For this review, take the finished solid that the model builds, in its own axes (mm). Coordinates: 2 decimals unless noted, no trailing zeros. Write each loop counter-clockwise with the first axis right and the second up, starting at its lowest first coordinate (ties: lowest second). Pieces come first, ordered by that corner, then holes. Notation, with made-up numbers: M -23.5,88 L 8.5,88 A15 cw 8.5,111 Z; hole C 4,-30.5 d2. An arc over 180 degrees is marked long. One line per question, with ' | ' between items.
from build123d import *

# Parameters (mm, degrees)
SKETCH1_R                                      = 1.7
BOSS_EXTRUDE1_DEPTH                            = 1.5875
SKETCH2_R                                      = 9
CUT_EXTRUDE1_DEPTH                             = 2.5875
CSK_FOR_M3_FLAT_HEAD_MACHINE_SCREW1_AT_2_COUNT = 2
CSK_FOR_M3_FLAT_HEAD_MACHINE_SCREW1_AT_2_PITCH = 11.799694945
CSK_FOR_M3_FLAT_HEAD_MACHINE_SCREW1_AT_3_COUNT = 2
CSK_FOR_M3_FLAT_HEAD_MACHINE_SCREW1_AT_3_PITCH = 38.059706694
CSK_FOR_M3_FLAT_HEAD_MACHINE_SCREW1_AT_4_COUNT = 2
CSK_FOR_M3_FLAT_HEAD_MACHINE_SCREW1_AT_4_PITCH = 65.441137915
CSK_FOR_M3_FLAT_HEAD_MACHINE_SCREW1_AT_5_COUNT = 2
CSK_FOR_M3_FLAT_HEAD_MACHINE_SCREW1_AT_5_PITCH = 98.21142491
CSK_FOR_M3_FLAT_HEAD_MACHINE_SCREW1_AT_6_COUNT = 2
CSK_FOR_M3_FLAT_HEAD_MACHINE_SCREW1_AT_6_PITCH = 136.991721698
CSK_FOR_M3_FLAT_HEAD_MACHINE_SCREW1_AT_7_COUNT = 2
CSK_FOR_M3_FLAT_HEAD_MACHINE_SCREW1_AT_7_PITCH = 176.317837002
CSK_FOR_M3_FLAT_HEAD_MACHINE_SCREW1_AT_8_COUNT = 2
CSK_FOR_M3_FLAT_HEAD_MACHINE_SCREW1_AT_8_PITCH = 185.829698762
CSK_FOR_M3_FLAT_HEAD_MACHINE_SCREW1_AT_9_COUNT = 2
CSK_FOR_M3_FLAT_HEAD_MACHINE_SCREW1_AT_9_PITCH = 185.066161853
CSK_FOR_M3_FLAT_HEAD_MACHINE_SCREW1_AT_1_COUNT = 2
CSK_FOR_M3_FLAT_HEAD_MACHINE_SCREW1_AT_1_PITCH = 174.805587361
CSK_FOR_M3_FLAT_HEAD_MACHINE_SCREW1_2_COUNT    = 2
CSK_FOR_M3_FLAT_HEAD_MACHINE_SCREW1_2_PITCH    = 135.039792437
CSK_FOR_M3_FLAT_HEAD_MACHINE_SCREW1_3_COUNT    = 2
CSK_FOR_M3_FLAT_HEAD_MACHINE_SCREW1_3_PITCH    = 95.46987855
CSK_FOR_M3_FLAT_HEAD_MACHINE_SCREW1_4_COUNT    = 2
CSK_FOR_M3_FLAT_HEAD_MACHINE_SCREW1_4_PITCH    = 62.253136917
CSK_FOR_M3_FLAT_HEAD_MACHINE_SCREW1_5_COUNT    = 2
CSK_FOR_M3_FLAT_HEAD_MACHINE_SCREW1_5_PITCH    = 32.271532316


with BuildPart() as part:
    # Sketch1 → Boss-Extrude1 (new body)
    with BuildSketch(Plane.XY):
        with BuildLine():
            Line((-21.913942314, 59.552395428), (-102.015642796, 95.25964371))
            ThreePointArc((-102.015642796, 95.25964371), (-106.983028684, 96.085831021), (-111.723245825, 94.386463641))
            Line((-111.723245825, 94.386463641), (-171.498000771, 121.032489918))
            ThreePointArc((-171.498000771, 121.032489918), (-198.238379477, 110.781775471), (-187.98766503, 84.041396765))
            Line((-187.98766503, 84.041396765), (-128.212910083, 57.395370488))
            ThreePointArc((-128.212910083, 57.395370488), (-126.308202352, 52.73386896), (-122.373252992, 49.591627472))
            Line((-122.373252992, 49.591627472), (-42.27155251, 13.884379189))
            ThreePointArc((-42.27155251, 13.884379189), (-34.620598521, 13.6805488), (-29.066427223, 18.946460398))
            Line((-29.066427223, 18.946460398), (-16.851861106, 46.347270141))
            ThreePointArc((-16.851861106, 46.347270141), (-16.648030717, 53.99822413), (-21.913942314, 59.552395428))
        make_face()
        with Locations((-99.517086056, 91.408706914)):
            Circle(SKETCH1_R, mode=Mode.SUBTRACT)
        with Locations((-62.982673065, 75.122618757)):
            Circle(SKETCH1_R, mode=Mode.SUBTRACT)
        with Locations((-26.448260075, 58.836530601)):
            Circle(SKETCH1_R, mode=Mode.SUBTRACT)
        with Locations((-20.722062659, 44.787930558)):
            Circle(SKETCH1_R, mode=Mode.SUBTRACT)
        with Locations((-30.493715553, 22.867282764)):
            Circle(SKETCH1_R, mode=Mode.SUBTRACT)
        with Locations((-44.77010925, 17.735315986)):
            Circle(SKETCH1_R, mode=Mode.SUBTRACT)
        with Locations((-81.304522241, 34.021404143)):
            Circle(SKETCH1_R, mode=Mode.SUBTRACT)
        with Locations((-117.838935231, 50.307492299)):
            Circle(SKETCH1_R, mode=Mode.SUBTRACT)
        with Locations((-131.618242769, 99.970559768)):
            Circle(SKETCH1_R, mode=Mode.SUBTRACT)
        with Locations((-145.664993804, 68.459628564)):
            Circle(SKETCH1_R, mode=Mode.SUBTRACT)
        with Locations((-173.979163871, 81.081346885)):
            Circle(SKETCH1_R, mode=Mode.SUBTRACT)
        with Locations((-159.932412836, 112.592278089)):
            Circle(SKETCH1_R, mode=Mode.SUBTRACT)
        with Locations((-192.145991763, 114.525444092)):
            Circle(SKETCH1_R, mode=Mode.SUBTRACT)
        with Locations((-196.950263565, 103.748070885)):
            Circle(SKETCH1_R, mode=Mode.SUBTRACT)
    extrude(amount=BOSS_EXTRUDE1_DEPTH)

    # Sketch2 → Cut-Extrude1 (cut, through all)
    with BuildSketch(Plane(origin=(0, 0, 0), x_dir=(-1, 0, 0), z_dir=(0, 0, -1))):
        with Locations((179.7428329, 102.536943342)):
            Circle(SKETCH2_R)
    extrude(amount=-CUT_EXTRUDE1_DEPTH, mode=Mode.SUBTRACT)

    # Sketch3 → CSK for M3 Flat Head Machine Screw1 (revolve, cut)
    with BuildSketch(Plane(origin=(-192.145991763, 114.525444092, 1.5875), x_dir=(0, -1, 0), z_dir=(1, 0, 0))):
        Polygon((0, 0), (0, 1.5875), (1.7, 1.5875), (1.7, 1.45), (3.15, 0), align=None)
    csk_for_m3_flat_head_machine_screw1 = revolve(axis=Axis((-192.145991763, 114.525444092, 7.9375), (0, 0, -1)), mode=Mode.SUBTRACT)

    # CSK for M3 Flat Head Machine Screw1 at 2: CSK for M3 Flat Head Machine Screw1 ×2
    with Locations(*[Vector(-0.407152204, -0.913360325, 0) * (i * CSK_FOR_M3_FLAT_HEAD_MACHINE_SCREW1_AT_2_PITCH) for i in range(1, CSK_FOR_M3_FLAT_HEAD_MACHINE_SCREW1_AT_2_COUNT)]):
        add(csk_for_m3_flat_head_machine_screw1, mode=Mode.SUBTRACT)

    # CSK for M3 Flat Head Machine Screw1 at 3: CSK for M3 Flat Head Machine Screw1 ×2
    with Locations(*[Vector(0.477324432, -0.87872714, 0) * (i * CSK_FOR_M3_FLAT_HEAD_MACHINE_SCREW1_AT_3_PITCH) for i in range(1, CSK_FOR_M3_FLAT_HEAD_MACHINE_SCREW1_AT_3_COUNT)]):
        add(csk_for_m3_flat_head_machine_screw1, mode=Mode.SUBTRACT)

    # CSK for M3 Flat Head Machine Screw1 at 4: CSK for M3 Flat Head Machine Screw1 ×2
    with Locations(*[Vector(0.710271848, -0.703927483, 0) * (i * CSK_FOR_M3_FLAT_HEAD_MACHINE_SCREW1_AT_4_PITCH) for i in range(1, CSK_FOR_M3_FLAT_HEAD_MACHINE_SCREW1_AT_4_COUNT)]):
        add(csk_for_m3_flat_head_machine_screw1, mode=Mode.SUBTRACT)

    # CSK for M3 Flat Head Machine Screw1 at 5: CSK for M3 Flat Head Machine Screw1 ×2
    with Locations(*[Vector(0.756602978, -0.653874555, 0) * (i * CSK_FOR_M3_FLAT_HEAD_MACHINE_SCREW1_AT_5_PITCH) for i in range(1, CSK_FOR_M3_FLAT_HEAD_MACHINE_SCREW1_AT_5_COUNT)]):
        add(csk_for_m3_flat_head_machine_screw1, mode=Mode.SUBTRACT)

    # CSK for M3 Flat Head Machine Screw1 at 6: CSK for M3 Flat Head Machine Screw1 ×2
    with Locations(*[Vector(0.809110712, -0.587656239, 0) * (i * CSK_FOR_M3_FLAT_HEAD_MACHINE_SCREW1_AT_6_PITCH) for i in range(1, CSK_FOR_M3_FLAT_HEAD_MACHINE_SCREW1_AT_6_COUNT)]):
        add(csk_for_m3_flat_head_machine_screw1, mode=Mode.SUBTRACT)

    # CSK for M3 Flat Head Machine Screw1 at 7: CSK for M3 Flat Head Machine Screw1 ×2
    with Locations(*[Vector(0.835853508, -0.548952561, 0) * (i * CSK_FOR_M3_FLAT_HEAD_MACHINE_SCREW1_AT_7_PITCH) for i in range(1, CSK_FOR_M3_FLAT_HEAD_MACHINE_SCREW1_AT_7_COUNT)]):
        add(csk_for_m3_flat_head_machine_screw1, mode=Mode.SUBTRACT)

    # CSK for M3 Flat Head Machine Screw1 at 8: CSK for M3 Flat Head Machine Screw1 ×2
    with Locations(*[Vector(0.869894733, -0.493237421, 0) * (i * CSK_FOR_M3_FLAT_HEAD_MACHINE_SCREW1_AT_8_PITCH) for i in range(1, CSK_FOR_M3_FLAT_HEAD_MACHINE_SCREW1_AT_8_COUNT)]):
        add(csk_for_m3_flat_head_machine_screw1, mode=Mode.SUBTRACT)

    # CSK for M3 Flat Head Machine Screw1 at 9: CSK for M3 Flat Head Machine Screw1 ×2
    with Locations(*[Vector(0.926284564, -0.376824768, 0) * (i * CSK_FOR_M3_FLAT_HEAD_MACHINE_SCREW1_AT_9_PITCH) for i in range(1, CSK_FOR_M3_FLAT_HEAD_MACHINE_SCREW1_AT_9_COUNT)]):
        add(csk_for_m3_flat_head_machine_screw1, mode=Mode.SUBTRACT)

    # CSK for M3 Flat Head Machine Screw1 at 1: CSK for M3 Flat Head Machine Screw1 ×2
    with Locations(*[Vector(0.947897228, -0.318576279, 0) * (i * CSK_FOR_M3_FLAT_HEAD_MACHINE_SCREW1_AT_1_PITCH) for i in range(1, CSK_FOR_M3_FLAT_HEAD_MACHINE_SCREW1_AT_1_COUNT)]):
        add(csk_for_m3_flat_head_machine_screw1, mode=Mode.SUBTRACT)

    # CSK for M3 Flat Head Machine Screw1  2: CSK for M3 Flat Head Machine Screw1 ×2
    with Locations(*[Vector(0.956483392, -0.291786774, 0) * (i * CSK_FOR_M3_FLAT_HEAD_MACHINE_SCREW1_2_PITCH) for i in range(1, CSK_FOR_M3_FLAT_HEAD_MACHINE_SCREW1_2_COUNT)]):
        add(csk_for_m3_flat_head_machine_screw1, mode=Mode.SUBTRACT)

    # CSK for M3 Flat Head Machine Screw1  3: CSK for M3 Flat Head Machine Screw1 ×2
    with Locations(*[Vector(0.970242207, -0.242136447, 0) * (i * CSK_FOR_M3_FLAT_HEAD_MACHINE_SCREW1_3_PITCH) for i in range(1, CSK_FOR_M3_FLAT_HEAD_MACHINE_SCREW1_3_COUNT)]):
        add(csk_for_m3_flat_head_machine_screw1, mode=Mode.SUBTRACT)

    # CSK for M3 Flat Head Machine Screw1  4: CSK for M3 Flat Head Machine Screw1 ×2
    with Locations(*[Vector(0.972284322, -0.233801621, 0) * (i * CSK_FOR_M3_FLAT_HEAD_MACHINE_SCREW1_4_PITCH) for i in range(1, CSK_FOR_M3_FLAT_HEAD_MACHINE_SCREW1_4_COUNT)]):
        add(csk_for_m3_flat_head_machine_screw1, mode=Mode.SUBTRACT)

    # CSK for M3 Flat Head Machine Screw1  5: CSK for M3 Flat Head Machine Screw1 ×2
    with Locations(*[Vector(0.998204195, -0.059903136, 0) * (i * CSK_FOR_M3_FLAT_HEAD_MACHINE_SCREW1_5_PITCH) for i in range(1, CSK_FOR_M3_FLAT_HEAD_MACHINE_SCREW1_5_COUNT)]):
        add(csk_for_m3_flat_head_machine_screw1, mode=Mode.SUBTRACT)


solid = part.part
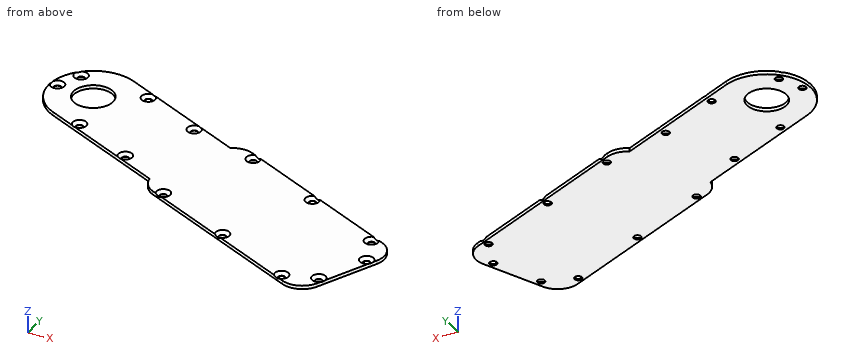
1. Take a section at C-C on x = -166.5. State the section outline as (y, z) points, plus the area to 3 significant figures.
Computed values:
outline: M 74.46,0 L 118.8,0 L 118.8,1.59 L 74.46,1.59 Z | area: 70.4 mm2
2. Clearance check with flat-ended pins moving along their axes: P1, Ø4, axis at x = -26.45, y = 58.84, coming from the +Z side; P2, Ø3, axis at x = -173.98, y = 81.08, coming from the +Z side; P3, Ø23.5, axis at x = -179.74, y = 102.54, coming from the +Z side; P4, Ø4.5, axis at x = -99.52, y = 91.41, coming from the +Z side. State where each tip first meets the part, or that it passes through.
Computed values:
P1: stops at z = 0.44 | P2: passes through | P3: stops at z = 1.59 | P4: stops at z = 0.69
3. Take a section at B-B on x = -56.5. State the section outline as (y, z) points.
Computed values:
outline: M 20.23,0 L 74.97,0 L 74.97,1.59 L 20.23,1.59 Z
4. Take a section at A-A on z = 0.45. Give the number of separate pieces and of enclosed holes in the cut face, plus the area to 3 significant figures.
Computed values:
separate pieces: 1 | enclosed holes: 15 | area: 8,110 mm2
5. For line 1 along X through (y, z) = (105, 1.4); line 2 along X through (y, z) = (109, 0.4); line 3 along Y through (x, z) = (-81, 1.15), list the stretches that pass through material, from the lowest coordinate up.
Computed values:
line 1: x = -199.84 to -199.64, -194.27 to -188.4, -171.09 to -135.53 | line 2: x = -198.93 to -186.01, -173.48 to -144.51 | line 3: y = 31.15 to 31.33, 36.72 to 85.89
